Geometry: final body of the model. Coordinates: model frame, mm. Give positions to 0.01 mm unless a question says otherwise; leave off trailing zeros. Order: outer loops, then holes, each group sorted by start corner. A loop starts at its lowest first (then second) coordinate and runs counter-clockwise, first axis right, second up. Notation, with made-up numbers: (26.25, 34) -> (40.25, 34) arc R13 cw to (40.25, 58) -> close; hole circle Ø1 at (18.25, 60). An arc over 180 degrees is marked (long way). One line per item, written item: value. Start each with the question number.
Autodesk Inventor part; units mm, degrees
ref_plane "YZ Plane" through (0, 0, 0) normal (1, 0, 0) x (0, 1, 0)
ref_plane "XZ Plane" through (0, 0, 0) normal (0, 1, 0) x (-1, 0, 0)
ref_plane "XY Plane" through (0, 0, 0) normal (0, 0, 1) x (1, 0, 0)
sketch "Sketch1" plane through (0, 0, 0) normal (1, 0, 0) x (0, 1, 0)
  line L0 (0, 0) -> (12, 0)
  line L1 (12, 0) -> (12, 12)
  line L2 (12, 12) -> (0, 12)
  line L3 (0, 12) -> (0, 0)
  line L4 (-1.5, 13.5) -> (13.5, 13.5)
  line L5 (13.5, 13.5) -> (13.5, -1.5)
  line L6 (13.5, -1.5) -> (-1.5, -1.5)
  line L7 (-1.5, -1.5) -> (-1.5, 13.5)
  dimension "d0" = 1.5
  dimension "d1" = 12
  dimension "d2" = 12
extrude "Extrusion1" add sketch "Sketch1" along normal blind 470
equation "\"d0\" = ZártSzelvényFalVastagság"
equation "\"d1\" = ZártSzelvényBelsőÁtmérő"
equation "\"d2\" = ZártSzelvényBelsőÁtmérő"
equation "\"ZártSzelvényFalVastagság\" = 1.5"
equation "\"ZártSzelvényBelsőÁtmérő\" = 12"
equation "\"CsapágyHázKülsőÁtmérő\" = 32"
equation "\"ZártSzelvényKülsőÁtmérő\" = 15"
equation "\"CsapágyBelsőÁtmérő\" = 12"
equation "\"CsapágyKülsőÁtmérő\" = 28"
equation "\"CsapágyHázBelsőÁtmérő\" = 26"
equation "\"CsapágyHázHoszza\" = 45"
equation "\"CsapágySzélesége\" = 8"
properties part number "KétvégenMartSzelvény" material "Acetal Resin, Black"
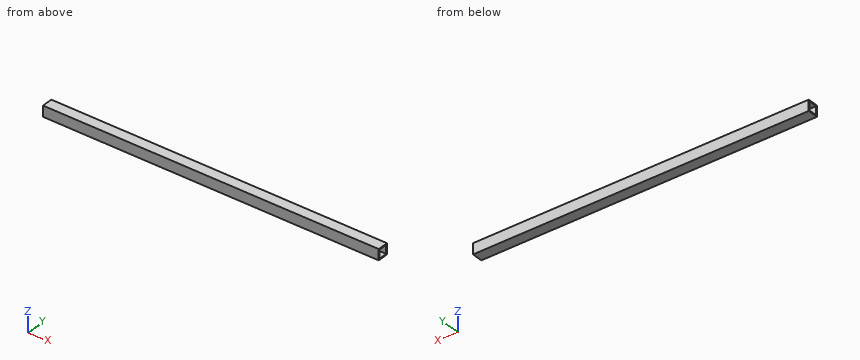
1. Material intervals for L1, parallel to Z at x = 122, y = 6.75, sorted ascending. Write a range as [from, to].
2. Cut plane A-A, the plane z = 6. Return loops of the section in (x, y).
3. Cut plane B-B, the plane x = 421.5. Return loops of the section in (y, z).
Answers follow:
1. L1: z = [-1.5, 0], [12, 13.5]
2. outline: (0, -1.5) -> (470, -1.5) -> (470, 0) -> (0, 0) -> close; (0, 12) -> (470, 12) -> (470, 13.5) -> (0, 13.5) -> close
3. outline: (-1.5, -1.5) -> (13.5, -1.5) -> (13.5, 13.5) -> (-1.5, 13.5) -> close; hole (0, 0) -> (12, 0) -> (12, 12) -> (0, 12) -> close
